Part model, mm, in its own coordinate system. Coordinates: 2 decimals unless noted, no trailing zeros. Write each loop counter-clockwise with the first axis right and the second up, starting at its lowest first coordinate (ties: lowest second). Pieces come first, ordered by that corner, then holes. Notation, with made-up numbers: (16, 44) -> (50, 44) arc R37 ccw to (50, 81) -> close; hole circle Ø1 at (-9, 77). An arc over 180 degrees is marked (long way). Write item = value, one per line.
Solid Edge part; units mm, degrees
sketch "Sketch1" plane through (0, 0, 0) normal (0, 0, 1) x (1, 0, 0)
  circle A0 centre (0, 0) radius 30
  circle A1 centre (0, 0) radius 8.5
extrude "Protrusion1" add sketch "Sketch1" along normal blind 2
sketch "Sketch2" plane through (0, 0, 0) normal (0, 0, 1) x (1, 0, 0)
  circle A0 centre (0, 11) radius 1.5
extrude "ExtrudedCutout_1" cut sketch "Sketch2" along normal mid plane 65.6802
pattern_circular "PatternOccurrence_1" count 6 over 360 about axis through (0, 0, 0) along (0, 0, -1) of "ExtrudedCutout_1"
sketch "Sketch3" plane through (0, 0, 0) normal (0, 0, 1) x (1, 0, 0)
  circle A0 centre (0, 25) radius 1.6
extrude "ExtrudedCutout_2" cut sketch "Sketch3" along normal mid plane 456.4322
pattern_circular "PatternOccurrence_2" count 4 over 360 about axis through (0, 0, 0) along (0, 0, -1) of "ExtrudedCutout_2"
Q1. Saw through at C-C on x = 25. Give the cut face in (y, z).
Model answer:
outline = (-16.58, 0) -> (-1.6, 0) -> (-1.6, 2) -> (-16.58, 2) -> close; (1.6, 0) -> (16.58, 0) -> (16.58, 2) -> (1.6, 2) -> close
Q2. Saw through at D-D on z = 1.4. Count the separate pieces of the cut face and the enclosed holes in it, and give its area (3 significant figures).
Model answer:
separate_pieces = 1
enclosed_holes = 11
area = 2,530 mm²
Q3. Probe line 1 (Y direction, x = 0, z = 0.6); line 2 (Y direction, x = 10.5, z = 1.7); line 3 (X direction, y = -25.5, z = 1). List the from-to ranges inside material, lowest first. Write a range as from..to.
Model answer:
line_1 = -30..-26.6, -23.4..-12.5, -9.5..-8.5, 8.5..9.5, 12.5..23.4, 26.6..30
line_2 = -28.1..-6.64, -4.36..4.36, 6.64..28.1
line_3 = -15.8..-1.52, 1.52..15.8
Q4. Saw through at B-B on x = 0. Give the cut face in (y, z).
Model answer:
outline = (-30, 0) -> (-26.6, 0) -> (-26.6, 2) -> (-30, 2) -> close; (-23.4, 0) -> (-12.5, 0) -> (-12.5, 2) -> (-23.4, 2) -> close; (-9.5, 0) -> (-8.5, 0) -> (-8.5, 2) -> (-9.5, 2) -> close; (8.5, 0) -> (9.5, 0) -> (9.5, 2) -> (8.5, 2) -> close; (12.5, 0) -> (23.4, 0) -> (23.4, 2) -> (12.5, 2) -> close; (26.6, 0) -> (30, 0) -> (30, 2) -> (26.6, 2) -> close
Q5. Saw through at A-A on y = 0. Give the cut face in (x, z), and give its area (3 significant figures).
Model answer:
outline = (-30, 0) -> (-26.6, 0) -> (-26.6, 2) -> (-30, 2) -> close; (-23.4, 0) -> (-8.5, 0) -> (-8.5, 2) -> (-23.4, 2) -> close; (8.5, 0) -> (23.4, 0) -> (23.4, 2) -> (8.5, 2) -> close; (26.6, 0) -> (30, 0) -> (30, 2) -> (26.6, 2) -> close
area = 73.2 mm²
Q6. Mould opens along Y. For faces 1 (the face through (-29.97, -1.32, 0.99)), 2 (the face through (6.2, -6.2, 0)), 3 (the face through (-23.414, -0.208, 0.986)), 4 (the face through (0.208, -23.414, 0.986)) say: released by +Y, released by -Y, zero draft, split by the parting line, or undercut.
Model answer:
face_1 = split by the parting line
face_2 = zero draft
face_3 = undercut
face_4 = undercut
